Geometry: see drawing. Coordinates: mm, zero at the bounding-box minimum. Coordinates: 2 decimals unless noted, no trailing zeros. Write each loop counter-clockwise with the first axis right and the second up, starting at its lowest first coordinate (ties: lowest second). Pieces come first, ordered by that corner, then holes. Notation, with made-up numbers: (0, 59) - (5, 59) arc R10 ccw to (5, 75) - close; hole circle Ø11 at (66, 76). An arc over 180 degrees is marked (long way). Use a Markdown table: item, result. Add a question column.
Q1. Material intervals for probe 1 along Z at (x, y) = (7.75, 6.5) (1 decimal); probe 2 along Y at (x, z) = (5.75, 10.5) (1 decimal); probe 3 along Z at (x, y) = (0.5, 7) (1 decimal), sorted ascending. Write a range as from..to.
Q2. Section query C-C (y = 6.35). Return the cut outline in (x, z) (1 decimal).
Q3. Section query B-B (z = 41). Return the cut outline in (x, y) (1 decimal), then the cut area to 3 significant figures.
Q4. Section query A-A (x = 3.5). Return the cut outline in (y, z), then the cut area to 3 significant figures.
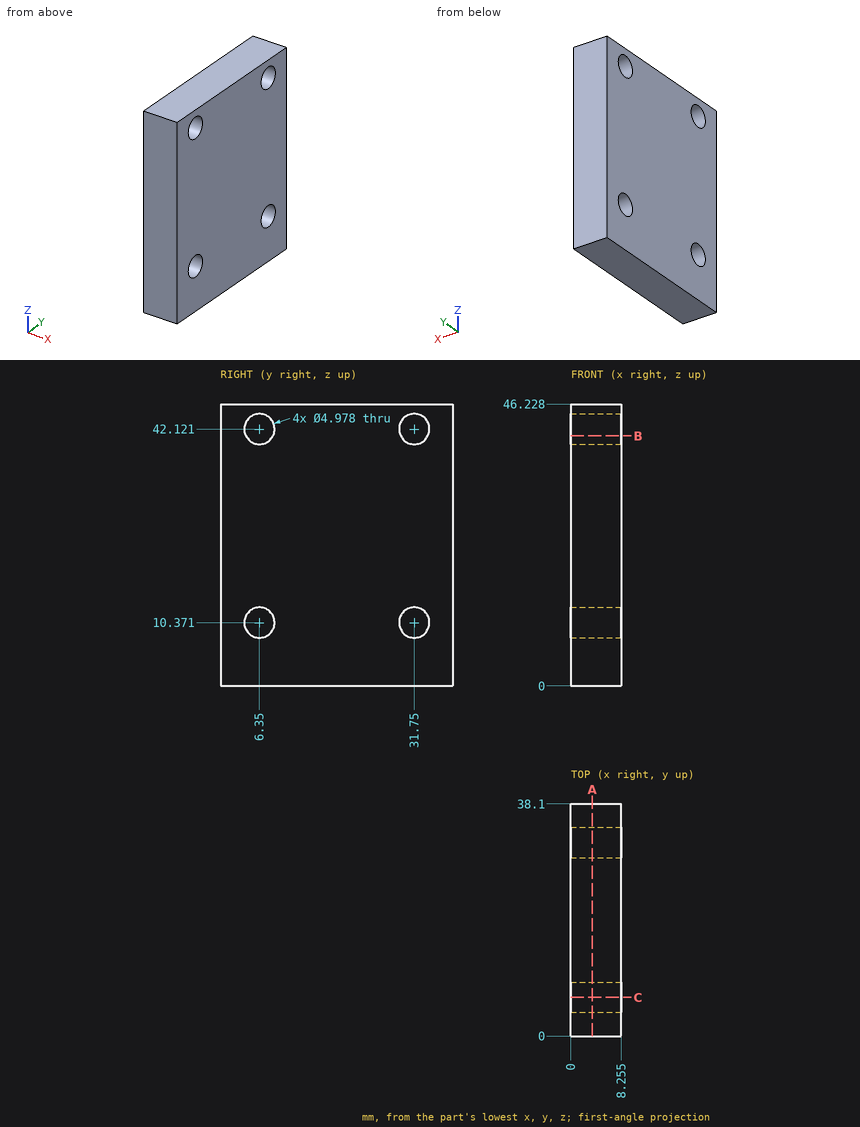
Values follow:
| question | item | result |
|---|---|---|
| 1 | probe 1 | 0..7.9, 12.9..39.6, 44.6..46.2 |
| 1 | probe 2 | 0..3.9, 8.8..29.3, 34.2..38.1 |
| 1 | probe 3 | 0..8, 12.8..39.7, 44.5..46.2 |
| 2 | outline | (0, 0) - (8.3, 0) - (8.3, 7.9) - (0, 7.9) - close; (0, 12.9) - (8.3, 12.9) - (8.3, 39.6) - (0, 39.6) - close; (0, 44.6) - (8.3, 44.6) - (8.3, 46.2) - (0, 46.2) - close |
| 3 | outline | (0, 0) - (8.3, 0) - (8.3, 4.1) - (0, 4.1) - close; (0, 8.6) - (8.3, 8.6) - (8.3, 29.5) - (0, 29.5) - close; (0, 34) - (8.3, 34) - (8.3, 38.1) - (0, 38.1) - close |
| 3 | area | 241 mm2 |
| 4 | outline | (0, 0) - (38.1, 0) - (38.1, 46.23) - (0, 46.23) - close; hole circle Ø4.98 at (6.35, 10.37); hole circle Ø4.98 at (6.35, 42.12); hole circle Ø4.98 at (31.75, 10.37); hole circle Ø4.98 at (31.75, 42.12) |
| 4 | area | 1,680 mm2 |
